```python
from build123d import *

# Parameters (mm, degrees)
F1_DEPTH = 28
F3_DEPTH = 2353
F5_DEPTH = 28
F6_R     = 2
F7_R     = 1
F8_R     = 4.25
F9_DEPTH = 25


with BuildPart() as f1:
    # F0 (on Top) → F1 (new body)
    with BuildSketch(Plane.XY):
        Polygon((-19.75, -17.750001), (-19.75, -19.75), (-9.25, -19.75), (19.75, 9.25), (19.75, 19.75), (17.750001, 19.75), (17.750001, 10.078427), (-10.078427, -17.750001), align=None)
    extrude(amount=F1_DEPTH)

    # F2 (on face) → F3 (join)
    with BuildSketch(Plane.XY.offset(28)):
        Polygon((-19.75, -19.75), (-9.25, -19.75), (19.75, 9.25), (19.75, 19.75), (11.25, 19.75), (11.25, 24.25), (9.25, 26.25), (9.25, 23.421573), (9.25, 19.75), (9.25, 17.750001), (17.750001, 17.750001), (17.750001, 10.078427), (16.585787, 8.914213), (-8.914213, -16.585787), (-10.078427, -17.750001), (-17.750001, -17.750001), (-17.750001, -9.25), (-19.75, -9.25), (-23.421573, -9.25), (-26.25, -9.25), (-24.25, -11.25), (-19.75, -11.25), align=None)
    extrude(amount=F3_DEPTH)

    # F4 (on face) → F5 (join)
    with BuildSketch(Plane.XY.offset(2381)):
        Polygon((19.75, 9.25), (19.75, 19.75), (17.750001, 19.75), (17.750001, 10.078427), (-10.078427, -17.750001), (-19.75, -17.750001), (-19.75, -19.75), (-9.25, -19.75), align=None)
    extrude(amount=F5_DEPTH)

    # F6
    f6_edges = [f1.edges().sort_by_distance(p)[0] for p in [
        (19.75, 9.25, 1204.5),
        (-9.25, -19.75, 1204.5),
    ]]
    fillet(f6_edges, radius=F6_R)

    # F7
    f7_edges = [f1.edges().sort_by_distance(p)[0] for p in [
        (-19.75, -19.75, 1204.5),
        (19.75, 19.75, 1204.5),
    ]]
    fillet(f7_edges, radius=F7_R)

    # F8 (on face) → F9 (cut)
    with BuildSketch(Plane(origin=(3.835787, -3.835787, 0), x_dir=(-0.707107, -0.707107, 0), z_dir=(-0.707107, 0.707107, 0))):
        with Locations((0, 14)):
            Circle(F8_R)
    extrude(amount=-F9_DEPTH, mode=Mode.SUBTRACT)


solid = f1.part
```
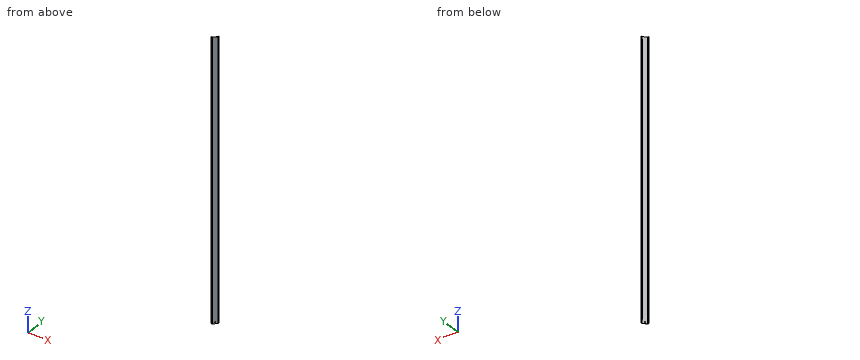
The listing builds one solid part. Answer for the finished solid, in the listing's coordinates (mm). Give positions to 0.01 mm unless a question says otherwise; leave off trailing zeros. Loops run counter-clockwise (first coordinate to the right, second up) from the corner with the lowest first, then second, coordinate; pieces in that order, holes last. Notation, with made-up numbers: (-10.75, -34) - (35.25, -34) arc R17 ccw to (35.25, -25) - close; hole circle Ø3 at (72.25, 60). An arc over 180 degrees is marked (long way). Return JSON: item names as keys, results as strings. Group by question number.
1. Straight lines are drawn through the part: line 1 (X direction, y = 13, z = 1478.5); line 2 (Z direction, x = -18, y = -10.5); line 3 (X direction, y = -15.5, z = 1424.5). For each, find the intervals that lie inside material, in ascending order. Write a range as [from, to].
2. Find section A-A (z = 1373). Write down the section's boundary in (x, y), then the cut area to 3 significant figures.
3. Given pin 1 Ø4 at (y, z) = (-14, 492) entering from -X; pin 2 Ø2.5 at (y, z) = (-12, 1633) entering from +X; pin 3 Ø8 at (x, z) = (-10.5, 832) entering from +Y; pin 4 Ø9.5 at (x, y) = (-22.5, -14.5) entering from +Z, each flat-ended and moving along its own axis, determine where each tip first touches the part or whether it passes through.
Verdict:
{
 "1": {"line 1": "x = [17.75, 19.75]", "line 2": "z = [28, 2381]", "line 3": "x = [-19.75, -17.75], [-7.83, -5]"},
 "2": {"outline": "(-26.25, -9.25) - (-24.25, -11.25) - (-19.75, -11.25) - (-19.75, -18.75) arc R1 ccw to (-18.75, -19.75) - (-10.08, -19.75) arc R2 ccw to (-8.66, -19.16) - (19.16, 8.66) arc R2 ccw to (19.75, 10.08) - (19.75, 18.75) arc R1 ccw to (18.75, 19.75) - (11.25, 19.75) - (11.25, 24.25) - (9.25, 26.25) - (9.25, 17.75) - (17.75, 17.75) - (17.75, 10.08) - (-10.08, -17.75) - (-17.75, -17.75) - (-17.75, -9.25) - close", "area": "176 mm^2"},
 "3": {"pin 1": "stops at x = -19.75", "pin 2": "stops at x = -0.25", "pin 3": "stops at y = -14.17", "pin 4": "stops at z = 2409"}
}
